Read the model definition and answer for the solid it produces. Units are mm, in the model's axes. A direction names the side the tool comes from. Give positions to 0.01 mm unless a question says otherwise; leave off trailing zeros. Loops run counter-clockwise (first coordinate to the right, second up) from the corner with the lowest first, then second, coordinate; pieces in that order, holes last. Notation, with made-up numbers: (59.5, -5) - (96.5, -5) arc R26 cw to (96.5, 34) - close; hole circle Ø3 at (42, 30.25). An arc over 180 degrees is marked (long way). Use a Markdown table: item, result. Add a question column.
Item 1: This flat-tipped pin is pushed along its axis until it touches: P1, Ø1, axis at x = -1, z = 0.5, coming from the +Y side. Where does it stop, or does it pass through?
Item 2: Which of the six approach directions +Z, -Z, +X, -X, +Y, -Y give full straight-line access (tool end or side, diameter ignored) to faces 1 (the face through (0, -35, 0)), 2 (the face through (-0.372, -15.773, -0.485))?
Item 3: A cutting plane is placed at B-B (y = -9.5). Determine the outline of the cut face in (x, z), plus the area to 3 significant figures.
Item 4: Consider probe 1 along Y at (x, z) = (-0.7, 0.5); probe 2 along Z at (x, y) = (-0.4, -13); probe 3 along Z at (x, y) = (0.55, -28). Determine where each line is inside the solid, lowest interval first. Write a range as [from, to].
Item 5: A cutting plane is placed at A-A (z = 0). Determine the outline of the cut face in (x, y).
from build123d import *

# Parameters (mm, degrees)
BOSS_EXTRUDE3_DEPTH      = 4
BOSS_EXTRUDE3_DEPTH_BACK = 50
SKETCH2_R                = 0.611392816
BOSS_EXTRUDE4_DEPTH      = 0.5
SKETCH4_W                = 4.000836521
SKETCH4_H                = 3.633574568
CUT_EXTRUDE1_DEPTH       = 15


with BuildPart() as part:
    # Sketch2 → Boss-Extrude3 (new, two sides: drawn at the far end of the back side and taken through both)
    with BuildSketch(Plane(origin=(0, 0, 0), x_dir=(1, 0, 0), z_dir=(0, 1, 0)).offset(-BOSS_EXTRUDE3_DEPTH_BACK)):
        with Locations(Location((0, 0, 0), (0, 0, 270))):
            Circle(SKETCH2_R)
    extrude(amount=BOSS_EXTRUDE3_DEPTH + BOSS_EXTRUDE3_DEPTH_BACK)

    # Sketch3 → Boss-Extrude4 (add)
    with BuildSketch(Plane(origin=(0, 4, 0), x_dir=(1, 0, 0), z_dir=(0, 1, 0))):
        Polygon((0.842464754, -0.774154905), (1.091670191, 0.342518427), (0.249205437, 1.116673331), (-0.842464754, 0.774154905), (-1.091670191, -0.342518427), (-0.249205437, -1.116673331), align=None)
    extrude(amount=BOSS_EXTRUDE4_DEPTH)

    # Sketch4 → Cut-Extrude1 (cut)
    with BuildSketch(Plane(origin=(0, -50, 0), x_dir=(-1, 0, 0), z_dir=(0, -1, 0))):
        with Locations((-0.863813315, -0.094243853)):
            Rectangle(SKETCH4_W, SKETCH4_H)
    extrude(amount=-CUT_EXTRUDE1_DEPTH, mode=Mode.SUBTRACT)


solid = part.part
Geometry says:
| question | item | result |
|---|---|---|
| 1 | P1 | y = 4.5 |
| 2 | face 1 | +Z, -Z, +X, -X, -Y |
| 2 | face 2 | -Y |
| 3 | outline | circle Ø1.22 at (0, 0) |
| 3 | area | 1.17 mm² |
| 4 | probe 1 | [4, 4.5] |
| 4 | probe 2 | [-0.46, 0.46] |
| 4 | probe 3 | [-0.27, 0.27] |
| 5 | outline | (-1.02, 4) - (-0.61, 4) - (-0.61, -35) - (0.61, -35) - (0.61, 4) - (1.02, 4) - (1.02, 4.5) - (-1.02, 4.5) - close |
